from build123d import *

# Parameters (mm, degrees)
CROQUIS1_W              = 130
CROQUIS1_H              = 3
SALIENTE_EXTRUIR1_DEPTH = 3


with BuildPart() as part:
    # Croquis1 → Saliente-Extruir1 (new body)
    with BuildSketch(Plane(origin=(0, 0, 0), x_dir=(0, 0, -1), z_dir=(1, 0, 0))):
        Polygon((-80.00000142, -80), (-80.00000142, -90), (-77.00000142, -90), (-77.000027229, -100), (-80, -100), (-80, -250), (-1.5, -250), (-1.5, -210), (1.5, -210), (1.5, -250), (80, -250), (80, -100), (77.000027229, -100), (77.00000142, -90), (80.00000142, -90), (80.00000142, -80), (77.000019468, -80), (77.000001401, -70.000000014), (80.000001401, -70.000000014), (80.000001401, -60.000000014), (77.000019449, -60.000000014), (77.000001383, -50.000000028), (80.000001383, -50.000000028), (80.000001383, -40.000000028), (77.000019431, -40.000000028), (77.000001365, -30.000000042), (80.000001365, -30.000000042), (80.000001365, -20.000000042), (77.000019412, -20.000000042), (77.000001346, -10.000000056), (80.000001346, -10.000000056), (80.000001346, -5.6e-08), (77.000019394, -5.6e-08), (77.000001328, 9.99999993), (80.000001328, 9.99999993), (80.000001328, 19.99999993), (77.000019376, 19.99999993), (77.00000131, 29.999999916), (80.00000131, 29.999999916), (80.00000131, 39.999999916), (77.000019357, 39.999999916), (77.000001291, 49.999999903), (80.000001291, 49.999999903), (80.000001291, 59.999999903), (77.000019339, 59.999999903), (77.000001273, 69.999999889), (80.000001273, 69.999999889), (80.000001273, 79.999999889), (77.000019321, 79.999999889), (77.000001254, 90), (80, 90), (80, 97), (80, 100), (70, 100), (70, 97), (60, 97), (60, 100), (50, 100), (50, 97), (40, 97), (40, 100), (30, 100), (30, 97), (20, 97), (20, 100), (10, 100), (10, 97), (0, 97), (0, 100), (-10, 100), (-10, 97), (-20, 97), (-20, 100), (-30, 100), (-30, 97), (-40, 97), (-40, 100), (-50, 100), (-50, 97), (-60, 97), (-60, 100), (-70, 100), (-70, 97), (-80, 97), (-80, 90), (-77.000001254, 90), (-77.000019321, 79.999999889), (-80.000001273, 79.999999889), (-80.000001273, 69.999999889), (-77.000001273, 69.999999889), (-77.000019339, 59.999999903), (-80.000001291, 59.999999903), (-80.000001291, 49.999999903), (-77.000001291, 49.999999903), (-77.000019357, 39.999999916), (-80.00000131, 39.999999916), (-80.00000131, 29.999999916), (-77.00000131, 29.999999916), (-77.000019376, 19.99999993), (-80.000001328, 19.99999993), (-80.000001328, 9.99999993), (-77.000001328, 9.99999993), (-77.000019394, -5.6e-08), (-80.000001346, -5.6e-08), (-80.000001346, -10.000000056), (-77.000001346, -10.000000056), (-77.000019412, -20.000000042), (-80.000001365, -20.000000042), (-80.000001365, -30.000000042), (-77.000001365, -30.000000042), (-77.000019431, -40.000000028), (-80.000001383, -40.000000028), (-80.000001383, -50.000000028), (-77.000001383, -50.000000028), (-77.000019449, -60.000000014), (-80.000001401, -60.000000014), (-80.000001401, -70.000000014), (-77.000001401, -70.000000014), (-77.000019468, -80), align=None)
        with Locations((0, -98.5)):
            Rectangle(CROQUIS1_W, CROQUIS1_H, mode=Mode.SUBTRACT)
    extrude(amount=SALIENTE_EXTRUIR1_DEPTH)


solid = part.part
The listing builds one solid part. Answer for the finished solid, in the listing's coordinates (mm). Coordinates: 2 decimals unless noted, no trailing zeros. Order: outer loops, then holes, each group sorted by start corner. A loop starts at its lowest first (then second) coordinate and runs counter-clockwise, first axis right, second up.
Q1. Consider line 1 (Y direction, x = 2.6, z = -6); line 2 (Z direction, x = 2.2, y = -218.5); line 3 (Z direction, x = 0.7, y = -55.5). Determine where each line is inside the solid, lowest interval first.
Q2. Given P1, Ø0.9, axis at x = 1, z = 76, coming from the +Y side; P2, Ø12, axis at y = -83, z = 0, coming from the -X side; P3, Ø0.9, axis at x = 1, y = 67, coming from the -Z side, each flat-ended and moving along its own axis, determine where each tip first touches the part or whether it passes through.
Q3. A cutting plane is placed at A-A, the plane y = -226. Write down the section's boundary in (x, z), and give its area (3 significant figures).
Answers follow:
1. line 1: y = -250 to -100, -97 to 97
1. line 2: z = -80 to -1.5, 1.5 to 80
1. line 3: z = -77 to 77
2. P1: stops at y = 97
2. P2: stops at x = 0
2. P3: stops at z = -77
3. outline: (0, -80) - (3, -80) - (3, -1.5) - (0, -1.5) - close; (0, 1.5) - (3, 1.5) - (3, 80) - (0, 80) - close
3. area: 471 mm2
